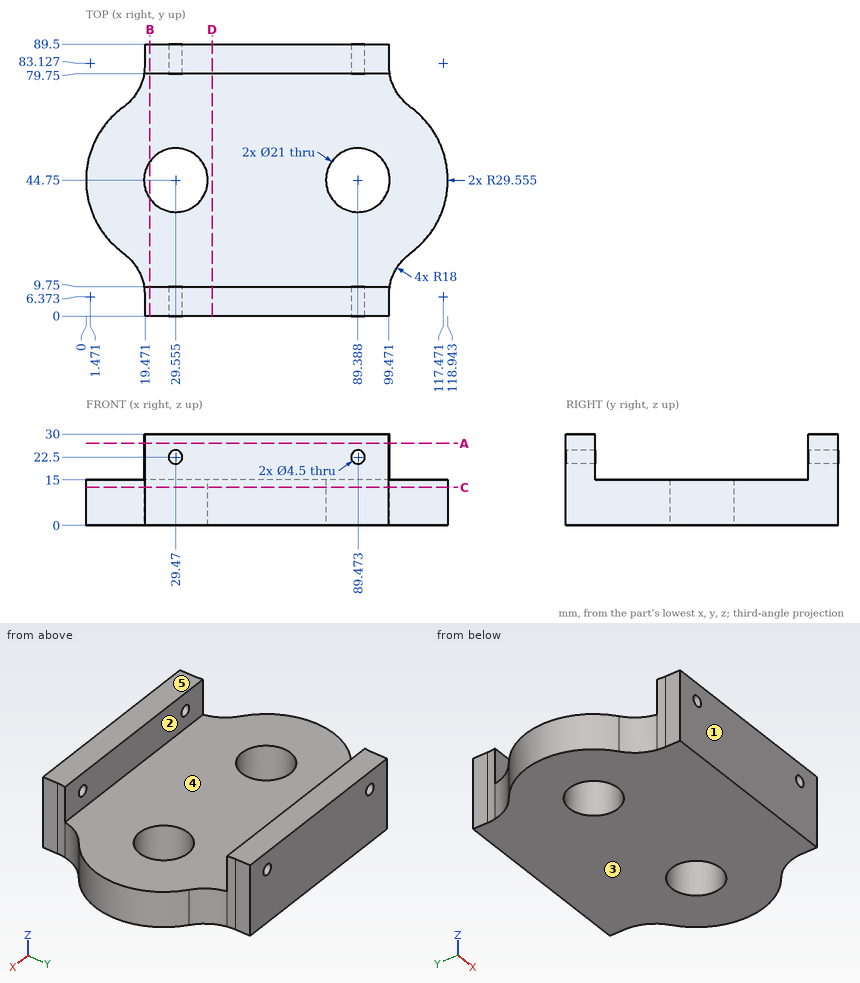
Geometry check sheet. Reference: drawing and pictorial views, mm from the part's lowest x, y, z. A direction names the side the tool comes from. Round coordinates to 2 decimals unless told otherwise and drop trailing zeros. Order: outer loops, then holes, each group sorted by start corner. A loop starts at its lowest first (then second) coordinate and runs counter-clockwise, first axis right, second up. Notation, with made-up numbers: M 22,69.25 L 44,69.25 A26 ccw 44,107.25 Z; hole C 8,79.25 d10. An arc over 180 degrees is marked long. One line per item, written item: value. Start each with the question number.
1. Section check D-D on x = 41.5. Enter the section's corners in (y, z).
2. Section check C-C on z = 12.5. Give the number of separate pieces and of enclosed holes in the cut face, and give its area (3 significant figures).
3. Gauge pin test, flat ends, axial feed: P1, Ø24, axis at x = 29.55, y = 44.75, coming from the +Z side; P2, Ø7, axis at y = 86.5, z = 10, coming from the +X side; P3, Ø6, axis at x = 29.47, z = 22.5, coming from the +Y side; P4, Ø5, axis at y = 2.5, z = 21.5, coming from the -X side. Record the tip position at first contact, or that the pin passes through.
4. Release check for a two-part mould opening along Y. For the marked faces 1, 2 and 3 record: released by +Y, released by -Y, zero draft, split by the parting line, or undercut.
5. Scan lines: line 1 along Y through (x, z) = (25, 26.75); line 2 along Y through (x, z) = (30, 7); line 3 along Z through (x, y) = (56.5, 75.5). Record each from-to range of solid material in increasing order.
6. Section check A-A on z = 27. Enter the section's corners in (x, y), and give its area (3 significant figures).
7. Access from +Z, -Z, +X, -X, +Y, -Y to the whole of each face (thin tool, end or side, straight path). Record for the marked faces 4 and 5.
8. Section check B-B on x = 21. Enter the section's corners in (y, z), and give its area (3 significant figures).
Results found:
1. outline: M 0,0 L 89.5,0 L 89.5,30 L 79.75,30 L 79.75,15 L 9.75,15 L 9.75,30 L 0,30 Z
2. separate pieces: 1
2. enclosed holes: 2
2. area: 8,110 mm^2
3. P1: z = 15
3. P2: x = 99.47
3. P3: y = 89.5
3. P4: x = 19.47
4. face 1: released by -Y
4. face 2: undercut
4. face 3: zero draft
5. line 1: 0 to 9.75, 79.75 to 89.5
5. line 2: 0 to 34.26, 55.24 to 89.5
5. line 3: 0 to 15
6. outline: M 19.15,9.75 A18 cw 19.47,6.37 L 19.47,0 L 99.47,0 L 99.47,6.37 A18 cw 99.79,9.75 Z; M 19.15,79.75 L 99.79,79.75 A18 cw 99.47,83.13 L 99.47,89.5 L 19.47,89.5 L 19.47,83.13 A18 cw Z
6. area: 1,560 mm^2
7. face 4: +Z, +X, -X
7. face 5: +Z, +X, -X, +Y, -Y
8. outline: M 0,0 L 38.66,0 L 38.66,15 L 9.75,15 L 9.75,30 L 0,30 Z; M 50.84,0 L 89.5,0 L 89.5,30 L 79.75,30 L 79.75,15 L 50.84,15 Z
8. area: 1,450 mm^2
